CAD build for the part. Positions are in the model's coordinates, mm. A direction names the side the tool comes from. Give positions to 0.01 mm unless a question says otherwise; leave off trailing zeros. Loops run counter-clockwise (first coordinate to the right, second up) from the corner with the lowest first, then second, coordinate; pieces in that order, holes last. Notation, with made-up numbers: M 15,79 L 30,79 A15 ccw 30,100 Z; hole C 72,2.5 d2. An arc over 180 degrees is marked long. Answer as CSV lines item,"result".
```python
from build123d import *

# Parameters (mm, degrees)
SKETCH1_W           = 39
SKETCH1_H           = 29.25
BOSS_EXTRUDE1_DEPTH = 3.25
SKETCH2_W           = 34
SKETCH2_H           = 24
CUT_EXTRUDE1_DEPTH  = 1
SKETCH3_W           = 34
SKETCH3_H           = 1.25
CUT_EXTRUDE2_DEPTH  = 1
SKETCH4_W           = 39
SKETCH4_H           = 22.75
BOSS_EXTRUDE2_DEPTH = 2.6
SKETCH6_W           = 34
SKETCH6_H           = 1.25
BOSS_EXTRUDE3_DEPTH = 1


with BuildPart() as part:
    # Sketch1 → Boss-Extrude1 (new body)
    with BuildSketch(Plane(origin=(0, 0, 0), x_dir=(1, 0, 0), z_dir=(0, 1, 0))):
        Rectangle(SKETCH1_W, SKETCH1_H)
    extrude(amount=BOSS_EXTRUDE1_DEPTH)

    # Sketch2 → Cut-Extrude1 (cut)
    with BuildSketch(Plane(origin=(0, 3.25, 0), x_dir=(1, 0, 0), z_dir=(0, 1, 0))):
        Rectangle(SKETCH2_W, SKETCH2_H)
    extrude(amount=-CUT_EXTRUDE1_DEPTH, mode=Mode.SUBTRACT)

    # Sketch3 → Cut-Extrude2 (cut)
    with BuildSketch(Plane(origin=(0, 3.25, 0), x_dir=(1, 0, 0), z_dir=(0, 1, 0))):
        with Locations((0, -12.625)):
            Rectangle(SKETCH3_W, SKETCH3_H)
    cut_extrude2 = extrude(amount=-CUT_EXTRUDE2_DEPTH, mode=Mode.SUBTRACT)

    # Mirror1: Cut-Extrude2 across plane
    add(cut_extrude2.mirror(Plane.XY), mode=Mode.SUBTRACT)

    # Sketch4 → Boss-Extrude2 (add)
    with BuildSketch(Plane.XY.offset(14.625)):
        with Locations((0, -11.375)):
            Rectangle(SKETCH4_W, SKETCH4_H)
    boss_extrude2 = extrude(amount=-BOSS_EXTRUDE2_DEPTH)

    # Sketch6 → Boss-Extrude3 (add)
    with BuildSketch(Plane.XZ.offset(22.75)):
        with Locations((0, 12.65)):
            Rectangle(SKETCH6_W, SKETCH6_H)
    boss_extrude3 = extrude(amount=BOSS_EXTRUDE3_DEPTH)

    # Mirror2: Boss-Extrude2, Boss-Extrude3 across plane
    add(boss_extrude2.mirror(Plane.XY))
    add(boss_extrude3.mirror(Plane.XY))


solid = part.part
```
Q1. Pin check, flat tips, straight feed: P1, Ø4, axis at x = -8.5, z = 7, coming from the -Y side; P2, Ø5, axis at x = -12, z = 7.5, coming from the +Y side; P3, Ø1.1, axis at x = 3.5, y = -23.5, coming from the -Z side (3 decimals). Stop position of each tip, or through.
Solution:
P1,"stops at y = 0"
P2,"stops at y = 2.25"
P3,"stops at z = -13.275"
Q2. Cut at D-D (x = 6). Write the cut outline in (y, z) (3 decimals).
Solution:
outline,"M -23.75,-13.275 L -22.75,-13.275 L -22.75,-14.625 L 3.25,-14.625 L 3.25,-13.25 L 2.25,-13.25 L 2.25,13.25 L 3.25,13.25 L 3.25,14.625 L -22.75,14.625 L -22.75,13.275 L -23.75,13.275 L -23.75,12.025 L 0,12.025 L 0,-12.025 L -23.75,-12.025 Z"
Q3. Cut at C-C (z = 8.75). Write the cut outline in (x, y).
Solution:
outline,"M -19.5,0 L 19.5,0 L 19.5,3.25 L 17,3.25 L 17,2.25 L -17,2.25 L -17,3.25 L -19.5,3.25 Z"
Q4. Wall check: line 1 (Z direction, x = -9.5, y = -10) (3 decimals); line 2 (Y direction, x = 18.5, z = -6.5); line 3 (Y direction, x = -15.5, z = 2.75). Give the ranges that are in metal, low to high. Write a range as [from, to].
Solution:
line 1,"z = [-14.625, -12.025], [12.025, 14.625]"
line 2,"y = [0, 3.25]"
line 3,"y = [0, 2.25]"
Q5. Cut at B-B (x = 17.5). Write the cut outline in (y, z) (3 decimals), and give its area (3 significant figures).
Solution:
outline,"M -22.75,-14.625 L 3.25,-14.625 L 3.25,14.625 L -22.75,14.625 L -22.75,12.025 L 0,12.025 L 0,-12.025 L -22.75,-12.025 Z"
area,"213 mm²"
Q6. Cut at A-A (y = -17.5). Write the cut outline in (x, z) (3 decimals), and give its area (3 significant figures).
Solution:
outline,"M -19.5,-14.625 L 19.5,-14.625 L 19.5,-12.025 L -19.5,-12.025 Z; M -19.5,12.025 L 19.5,12.025 L 19.5,14.625 L -19.5,14.625 Z"
area,"203 mm²"
Q7. Mould opens along X. For faces 1 (the flat face through (17, -23, -13)), 2 (the flat face through (17, 3, 0)), 3 (the flat face through (0, -12, -12.025)) say: released by +X, released by -X, zero draft, split by the parting line, or undercut.
Solution:
face 1,"released by +X"
face 2,"undercut"
face 3,"zero draft"
Q8. Which spindle directions (+Z, -Z, +X, -X, +Y, -Y) get a long thin tool onto all of the face, cutting with end or side? Do faces 4 (the flat face through (0, -23, 13.275)), 5 (the flat face through (0, 2.25, 0)), 6 (the flat face through (17, -23, 13)), 7 (the flat face through (-17, -23, -13)), 8 (the flat face through (0, -12, 12.025)). Say none if no direction does.
Solution:
face 4,"+Z, +X, -X, -Y"
face 5,"+Y"
face 6,"+Z, -Z, +X, -Y"
face 7,"+Z, -Z, -X, -Y"
face 8,"+X, -X, -Y"
